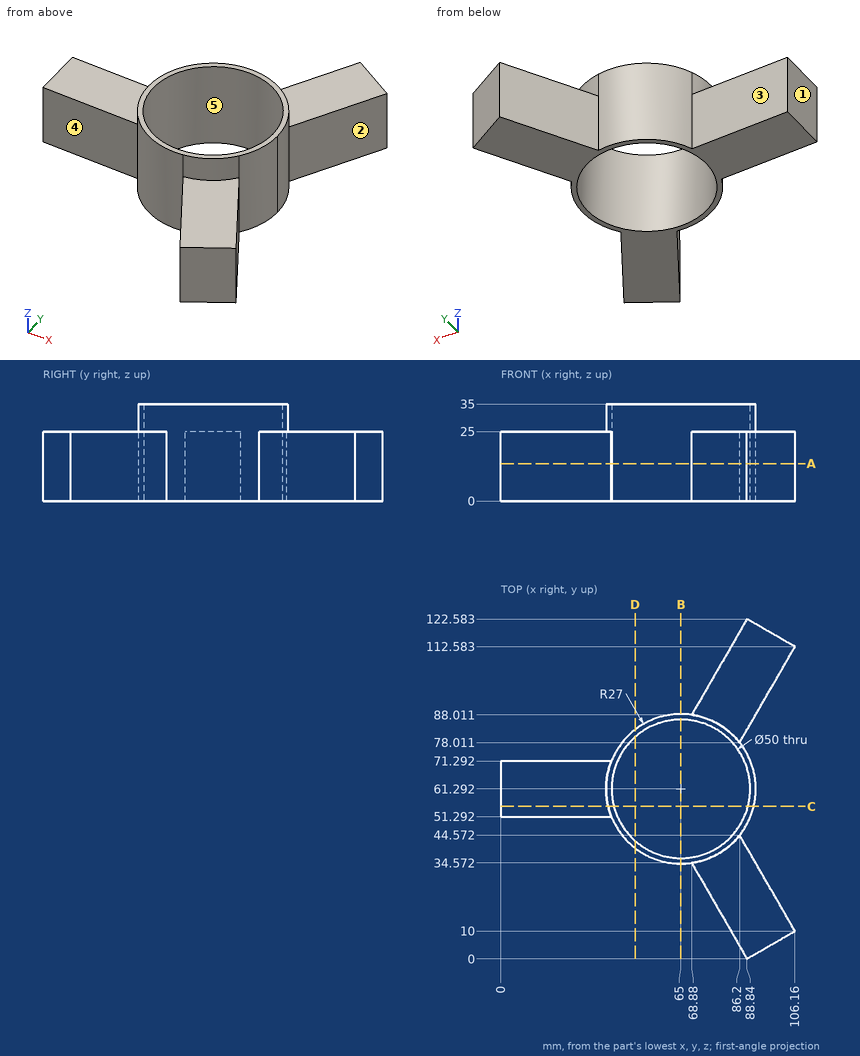
The figure shows three views and two pictorial views of one solid part (mm, origin at its lowest corner). Answer the questions. A direction names the side the tool comes from. Give positions to 0.01 mm unless a question says otherwise; leave off trailing zeros. Loops run counter-clockwise (first coordinate to the right, second up) from the corner with the lowest first, then second, coordinate; pieces in that order, holes last. Notation, with made-up numbers: (34.5, 15) - (85.5, 15) arc R35 ccw to (85.5, 50) - close; hole circle Ø5 at (-20, 72.25). An arc over 180 degrees is marked (long way). Use one line per item in the form item = value.
1. Section C-C on y = 55 is taken. Give the vertices of the cut face in (x, z) (1 decimal), then the cut area to 3 significant figures.
Calculated:
outline = (0, 0) - (40.8, 0) - (40.8, 35) - (38.7, 35) - (38.7, 25) - (0, 25) - close; (89.2, 0) - (91.3, 0) - (91.3, 35) - (89.2, 35) - close
area = 1,110 mm^2
2. Which of the six approach directions +Z, -Z, +X, -X, +Y, -Y give full straight-line access (tool end or side, diameter ignored) to the marked faces 1 and 2?
Calculated:
face_1 = +Z, -Z, -X, +Y, -Y
face_2 = +Z, -Z, +X
3. The mould has two halves that part along Y. Classify the marked faces 3, 4 and 5: pulls with the +Y half, pulls with the -Y half, needs draft (parallel to the pull), parting line crosses it, or undercut.
Calculated:
face_3 = pulls with the +Y half
face_4 = pulls with the -Y half
face_5 = undercut
4. Given pin 1 Ø18.5 at (x, y) = (85.5, 109.5) entering from +Z; pin 2 Ø10 at (x, z) = (81, 11.5) entering from -Y; pin 3 Ø7.5 at (x, z) = (26, 7) entering from -Y, each flat-ended and moving along its own axis, determine where each tip first touches the part or whether it passes through.
Calculated:
pin_1 = 25
pin_2 = 4.92
pin_3 = 51.29
5. Section A-A on z = 13.5 is taken. Give the vertices of the cut face in (x, y).
Calculated:
outline = (0, 51.29) - (39.92, 51.29) arc R27 ccw to (68.88, 34.57) - (88.84, 0) - (106.16, 10) - (86.2, 44.57) arc R27 ccw to (92, 61.29) arc R27 ccw to (86.2, 78.01) - (106.16, 112.58) - (88.84, 122.58) - (68.88, 88.01) arc R27 ccw to (39.92, 71.29) - (0, 71.29) - close; hole circle Ø50 at (65, 61.29)
6. Find the intervals of material crossed by line 1 along Y through (x, z) = (65, 24); line 2 along X through (y, z) = (73.5, 9) (1 decimal); line 3 along Z through (x, y) = (79, 18), in increasing order. Write a range as [from, to].
Calculated:
line_1 = [34.29, 36.29], [86.29, 88.29]
line_2 = [40.9, 43.2], [86.8, 89.1]
line_3 = [0, 25]
7. Section D-D on x = 48.5 is taken. Give the vertices of the cut face in (y, z).
Calculated:
outline = (39.92, 0) - (42.51, 0) - (42.51, 35) - (39.92, 35) - close; (80.07, 0) - (82.66, 0) - (82.66, 35) - (80.07, 35) - close
8. Section B-B on x = 65 is taken. Give the vertices of the cut face in (y, z).
Calculated:
outline = (34.29, 0) - (36.29, 0) - (36.29, 35) - (34.29, 35) - close; (86.29, 0) - (88.29, 0) - (88.29, 35) - (86.29, 35) - close
